Can you work these out from the model? Positions are in its coordinate system, mm. A direction names the side the tool comes from. Round coordinates to 2 decimals unless told otherwise and drop trailing zeros. Loops run counter-clockwise (first coordinate to the right, second up) from the corner with the lowest first, then second, coordinate; pieces in that order, holes last.
Autodesk Inventor part; units mm, degrees
ref_plane "YZ Plane" through (0, 0, 0) normal (1, 0, 0) x (0, 1, 0)
ref_plane "XZ Plane" through (0, 0, 0) normal (0, 1, 0) x (-1, 0, 0)
ref_plane "XY Plane" through (0, 0, 0) normal (0, 0, 1) x (1, 0, 0)
sketch "Skizze3" plane through (0, 0, 0) normal (0, 0, 1) x (1, 0, 0)
  line L0 (0, 0) -> (-120, 0)
  line L1 (-240, 0) -> (-240, 120)
  line L2 (-240, 120) -> (0, 120)
  line L3 (0, 120) -> (0, 0)
  line L4 (-248.2253, 60) -> (-229.9902, 60) construction
  line L5 (-189.05, 39.8483) -> (-189.05, 104.036) construction
  line L6 (-205.9145, 69.185) -> (-155.0384, 69.185) construction
  line L7 (-154.68, 50.3276) -> (-154.68, 100.4743) construction
  line L8 (-153.2541, 50.815) -> (-196.0103, 50.815) construction
  circle A0 centre (-180, 60) radius 3
  line L9 (-105, 40) -> (-80, 40)
  line L10 (-80, 40) -> (-80, 80)
  line L11 (-80, 80) -> (-105, 80)
  line L12 (-105, 80) -> (-105, 40)
  line L13 (-120, -37.5982) -> (-120, -22.8575) construction
  line L14 (-120, 0) -> (-240, 0)
  line L15 (-60, -24.367) -> (-60, 44.367) construction
  circle A1 centre (-180, 60) radius 20.5
  point P0 (-240, 60)
  point P1 (-189.05, 69.185)
  point P2 (-189.05, 50.815)
  point P3 (-154.68, 50.815)
  point P4 (-154.68, 69.185)
  point P5 (-105, 60)
  point P6 (-101.3, 43.7)
  point P7 (-230, 60)
  point P8 (-120, 120)
  point P9 (-180, 0)
  point P10 (-60, 0)
  point P11 (-60, 10)
  point P12 (-160, 10)
  point P13 (-160, 110)
  point P14 (-60, 110)
  point P15 (-60, 10)
  dimension "d4" = 120
  dimension "d5" = 240
  dimension "d6" = 60
  dimension "d8" = 9.05
  dimension "d9" = 34.37
  dimension "d11" = 9.185
  dimension "d12" = 18.37
  dimension "d17" = 6
  dimension "d18" = 40
  dimension "d19" = 25
  dimension "d20" = 75
  dimension "d21" = 3.7
  dimension "d22" = 3.7
  dimension "d39" = 10
  dimension "d40" = 10
  dimension "d41" = 10
  dimension "d42" = 10
  dimension "d43" = 10
  dimension "d51" = 80
  dimension "d52" = 80
  dimension "d53" = 41
extrude "Extrusion3" add sketch "Skizze3" against normal blind 5 contours L0 L14 L1 L2 L3 | L12 L11 L10 L9 | A1
hole "Bohrung1" at (-101.3, 43.7, 0) direction (0, 0, -1) diameter 2.459 end through all
pattern_linear "Rechteckige Anordnung1" count 2 spacing 32.6 along (0, 1, 0) count 2 spacing 27.6 along (1, 0, 0) of "Bohrung1"
fillet "Rundung1" radius 2 4 edges at (-240, 120, -2.5) (-240, 0, -2.5) (0, 120, -2.5) (0, 0, -2.5)
hole "Bohrung2" at (-230, 60, 0) at (-60, 10, 0) at (-160, 10, 0) at (-160, 110, 0) at (-60, 110, 0) direction (0, 0, -1) diameter 5.5 end through all
hole "Bohrung3" at (-189.05, 69.185, 0) at (-189.05, 50.815, 0) at (-154.68, 50.815, 0) at (-154.68, 69.185, 0) direction (0, 0, -1) diameter 2.7 end through all counterbore diameter 6 counterbore depth 3.2
equation "\"d34\" = d18 - 2 * d22"
properties part number "BT002_trajan20_21" material "Acryl"
(1) For faces 5 (the cylindrical face through (-227.315, 60.596, -2.535)), 6 (the flat face through (-188, 68, -3.2)), which set-ups out of +Z, -Z, +X, -X, +Y, -Y let a thin tool reach every point of the face, with its end or its side?
Worked answers:
face 5: +Z, -Z
face 6: +Z
(2) If we section it at A-A, the plane y = 60: List the corners of the cut face in (x, z) for me, then the cut area to 3 significant figures.
Worked answers:
outline: (-240, -5) - (-232.75, -5) - (-232.75, 0) - (-240, 0) - close; (-227.25, -5) - (-183, -5) - (-183, 0) - (-227.25, 0) - close; (-177, -5) - (0, -5) - (0, 0) - (-177, 0) - close
area: 1,140 mm2
(3) If we section it at B-B, the plane x = -180: List the corners of the cut face in (y, z) for me.
Worked answers:
outline: (0, -5) - (57, -5) - (57, 0) - (0, 0) - close; (63, -5) - (120, -5) - (120, 0) - (63, 0) - close
(4) Will these pins go through, and if not, where does the flat tip stop? P1, Ø6.5, axis at x = -60, y = 10, coming from the +Z side; P2, Ø5, axis at x = -154.68, y = 50.815, coming from the +Z side; P3, Ø4.5, axis at x = -230, y = 60, coming from the +Z side.
Worked answers:
P1: stops at z = 0
P2: stops at z = -3.2
P3: passes through
(5) If we mould it in two halves opening along X, with no side actions, what happens to faces 1 (the flat face through (-240, 59, -2)), 2 (the flat face through (-122, 120, -2)), 3 (the flat face through (0, 61, -2)), 4 (the cylindrical face through (-157.56, 8.73, -2.54))? For each: released by +X, released by -X, zero draft, split by the parting line, or undercut.
Worked answers:
face 1: released by -X
face 2: zero draft
face 3: released by +X
face 4: undercut
(6) If I drill on line 1 (Y direction, x = -101.3, z = -1.15); line 2 (X direction, y = 76.3, z = -2.15); line 3 (Y direction, x = -160, z = -3.6), over which ranges is the centre line in solid material (lowest first)?
Worked answers:
line 1: y = 0 to 42.47, 44.93 to 75.07, 77.53 to 120
line 2: x = -240 to -102.53, -100.07 to -74.93, -72.47 to 0
line 3: y = 0 to 7.25, 12.75 to 107.25, 112.75 to 120
